Design review of the part built by this model. Coordinates are the model's own, in mm. A direction names the side the tool comes from. Coordinates: 2 decimals unless noted, no trailing zeros. Write each loop counter-clockwise with the first axis right and the second up, starting at its lowest first coordinate (ties: lowest second). Pieces come first, ordered by that corner, then holes. Notation, with made-up numbers: (47, 12.5) -> (53, 12.5) arc R15 cw to (53, 17.5) -> close; hole circle Ø4 at (76.25, 7). An arc over 180 degrees is marked (long way). One line per question, with ' | ' between items. Start each with the question number.
Q1. Add section A-A on x = 37. State the section outline as (y, z) points, and give its area (3 significant figures).
Q2. Add section B-B on y = 10. State the section outline as (x, z) points (3 decimals).
Q3. For faces 4 (the flat face through (-80, 2, -5)), 5 (the cylindrical face through (102, 3, -4)), 6 (the flat face through (79, 2, 5)), list the 3-axis set-ups (+Z, -Z, +X, -X, +Y, -Y) from which the entire face can be reached by the end or side of a thin tool; tool diameter is ignored.
Q4. Wall thickness on probe 1 along X at (y, z) = (1.75, 0) (3 decimals); probe 2 along Y at (x, z) = (31.5, -9.5); probe 3 along Z at (x, y) = (6, 9): over which ranges is each line inside the solid? List them lowest first.
Q5. Draft analysis for pull direction Z (two halves, no side actions). For faces 1 (the cylindrical face through (-39.43, 2.46, 0.32)), 2 (the cylindrical face through (-4, 3, 102)), 3 (the flat face through (8, 0, -8)), state which applies: pulls with the +Z half, pulls with the -Z half, needs draft (parallel to the pull), parting line crosses it, or undercut.
Q6. For P1, Ø10, axis at x = -4, z = -82, coming from the +Y side; P2, Ø1.5, axis at y = 1.5, z = 85, coming from the +X side; P3, Ø3.5, axis at x = 99, z = 0, coming from the +Y side; P4, Ø5.5, axis at x = 75, y = 3.5, coming from the +Z side, all flat-tipped, find the tip position at first contact; note any pin that passes through.
Q7. Add section D-D on x = -57. State the section outline as (y, z) points.
Q8. Add section C-C on z = 20. State the section outline as (x, y) points.
from build123d import *

# Parameters (mm, degrees)
CROQUIS1_R              = 45
CROQUIS1_R_2            = 2.45
CROQUIS1_R_3            = 8.125
SALIENTE_EXTRUIR1_DEPTH = 5
CROQUIS1_2_R            = 12.125
CROQUIS1_2_R_2          = 8.125
EXTRUIR_L_MINA1_DEPTH   = 15
CROQUIS2_R              = 2.425
CORTAR_EXTRUIR2_DEPTH   = 3
CROQUIS3_W              = 59.27864045
CROQUIS3_H              = 10
CROQUIS3_R              = 2.05
CROQUIS3_W_2            = 10
CROQUIS3_H_2            = 59.27864045
SALIENTE_EXTRUIR2_DEPTH = 5
REDONDEO1_R             = 5
REDONDEO2_R             = 20


with BuildPart() as part:
    # Croquis1 → Saliente-Extruir1 (new body)
    with BuildSketch(Plane(origin=(0, 0, 0), x_dir=(1, 0, 0), z_dir=(0, 1, 0))):
        with Locations(Location((0, 0, 0), (0, 0, 270))):
            Circle(CROQUIS1_R)
        with Locations(Location((37, 0, 0), (0, 0, 270))):
            Circle(CROQUIS1_R_2, mode=Mode.SUBTRACT)
        with Locations(Location((-37, 0, 0), (0, 0, 90))):
            Circle(CROQUIS1_R_2, mode=Mode.SUBTRACT)
        with Locations(Location((0, 0, 0), (0, 0, 270))):
            Circle(CROQUIS1_R_3, mode=Mode.SUBTRACT)
    extrude(amount=SALIENTE_EXTRUIR1_DEPTH)

    # Croquis1<2> → Extruir-Lámina1 (add)
    with BuildSketch(Plane(origin=(0, 0, 0), x_dir=(1, 0, 0), z_dir=(0, 1, 0))):
        Circle(CROQUIS1_2_R)
        Circle(CROQUIS1_2_R_2, mode=Mode.SUBTRACT)
    extrude(amount=EXTRUIR_L_MINA1_DEPTH)

    # Croquis2 → Cortar-Extruir2 (cut)
    with BuildSketch(Plane(origin=(-12.125, 0, -11.125), x_dir=(0, 0, -1), z_dir=(1, 0, 0))):
        with Locations(Location((-11.125, 10, 0), (0, 0, 180))):
            Circle(CROQUIS2_R)
    extrude(amount=CORTAR_EXTRUIR2_DEPTH, mode=Mode.SUBTRACT)

    # Croquis3 → Saliente-Extruir2 (add)
    # profile 1 of 4: a face of its own
    with BuildSketch(Plane(origin=(0, 0, 0), x_dir=(1, 0, 0), z_dir=(0, 1, 0))):
        with Locations((74.360679775, 0)):
            Rectangle(CROQUIS3_W, CROQUIS3_H)
        with Locations(Location((99, 0, 0), (0, 0, 270))):
            Circle(CROQUIS3_R, mode=Mode.SUBTRACT)
    # profile 2 of 4: a face of its own
    with BuildSketch(Plane(origin=(0, 0, 0), x_dir=(1, 0, 0), z_dir=(0, 1, 0))):
        with Locations((0, 74.360679775)):
            Rectangle(CROQUIS3_W_2, CROQUIS3_H_2)
        with Locations(Location((0, 99, 0), (0, 0, 270))):
            Circle(CROQUIS3_R, mode=Mode.SUBTRACT)
    # profile 3 of 4: a face of its own
    with BuildSketch(Plane(origin=(0, 0, 0), x_dir=(1, 0, 0), z_dir=(0, 1, 0))):
        with Locations((0, -74.360679775)):
            Rectangle(CROQUIS3_W_2, CROQUIS3_H_2)
        with Locations(Location((0, -99, 0), (0, 0, 270))):
            Circle(CROQUIS3_R, mode=Mode.SUBTRACT)
    # profile 4 of 4: a face of its own
    with BuildSketch(Plane(origin=(0, 0, 0), x_dir=(1, 0, 0), z_dir=(0, 1, 0))):
        with Locations((-74.360679775, 0)):
            Rectangle(CROQUIS3_W, CROQUIS3_H)
        with Locations(Location((-99, 0, 0), (0, 0, 270))):
            Circle(CROQUIS3_R, mode=Mode.SUBTRACT)
    extrude(amount=SALIENTE_EXTRUIR2_DEPTH)

    # Redondeo1
    redondeo1_edges = [part.edges().sort_by_distance(p)[0] for p in [
        (5, 2.5, 104),
        (-5, 2.5, 104),
        (-104, 2.5, 5),
        (-104, 2.5, -5),
        (-5, 2.5, -104),
        (5, 2.5, -104),
        (104, 2.5, -5),
        (104, 2.5, 5),
    ]]
    fillet(redondeo1_edges, radius=REDONDEO1_R - 0.0001)  # a hair under: the kernel refuses the full size

    # Redondeo2
    redondeo2_edges = [part.edges().sort_by_distance(p)[0] for p in [
        (-5, 2.5, -44.72135955),
        (5, 2.5, -44.72135955),
        (44.72135955, 2.5, -5),
        (44.72135955, 2.5, 5),
        (5, 2.5, 44.72135955),
        (-5, 2.5, 44.72135955),
        (-44.72135955, 2.5, 5),
        (-44.72135955, 2.5, -5),
    ]]
    fillet(redondeo2_edges, radius=REDONDEO2_R)


solid = part.part
Output values:
1) outline: (0, -25.61) -> (5, -25.61) -> (5, -2.45) -> (0, -2.45) -> close; (0, 2.45) -> (5, 2.45) -> (5, 25.61) -> (0, 25.61) -> close | area: 232 mm2
2) outline: (-11.88, -2.425) arc R12.125 ccw (long way) to (-11.88, 2.425) -> (-9.125, 2.425) -> (-9.125, -2.425) -> close; hole circle Ø16.25 at (0, 0)
3) face 4: -Z, -X, +Y, -Y | face 5: -Z, +X, +Y, -Y | face 6: +Z, +X, +Y, -Y
4) probe 1: x = -104 to -101.05, -96.95 to -39.45, -34.55 to -8.125, 8.125 to 34.55, 39.45 to 96.95, 101.05 to 104 | probe 2: y = 0 to 5 | probe 3: z = -10.54 to -5.48, 5.48 to 10.54
5) face 1: undercut | face 2: pulls with the +Z half | face 3: needs draft
6) P1: stops at y = 5 | P2: stops at x = 5 | P3: passes through | P4: stops at z = 5
7) outline: (0, -5.23) -> (5, -5.23) -> (5, 5.23) -> (0, 5.23) -> close
8) outline: (-40.31, 0) -> (40.31, 0) -> (40.31, 5) -> (-40.31, 5) -> close
